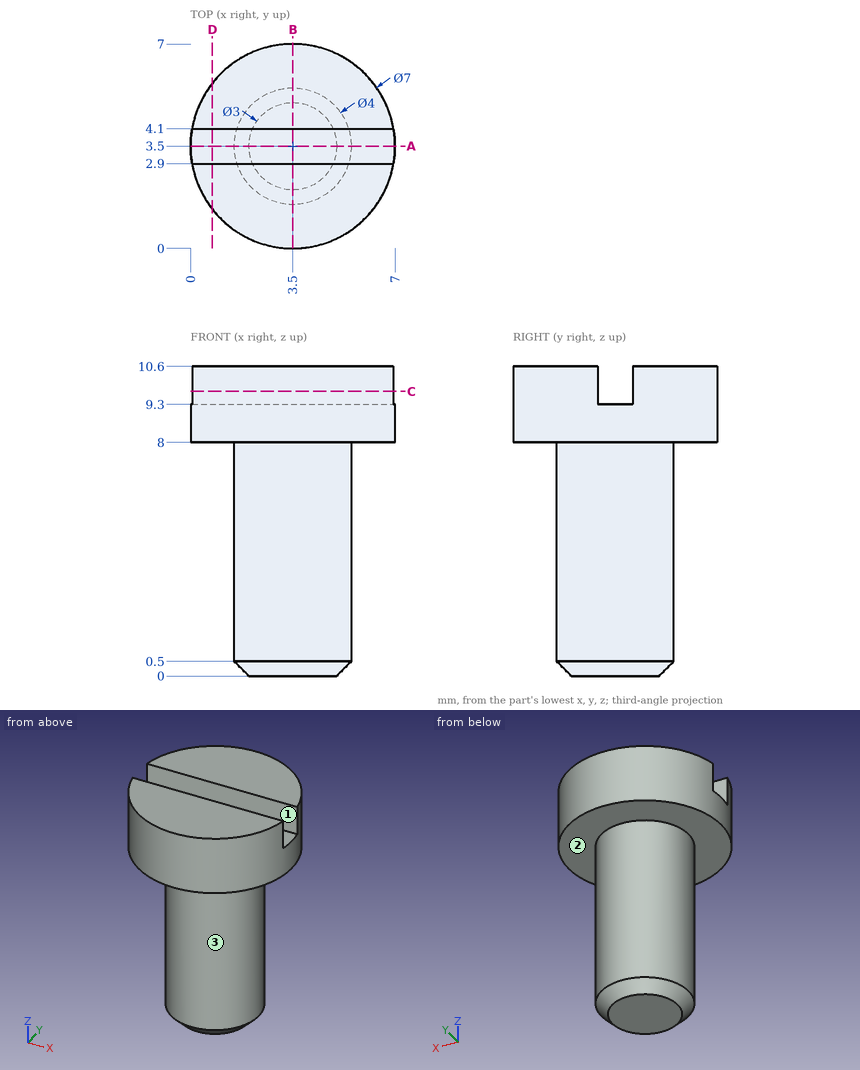
Job drawing, mm, ordinate dimensions from the low corner. One solid piece. Give positions to 0.01 mm unless a question says otherwise; leave off trailing zeros. Write each loop counter-clockwise with the first axis right and the second up, starting at its lowest first coordinate (ties: lowest second). Pieces come first, ordered by that corner, then holes. Notation, with made-up numbers: M -29,12 L -19,12 A35 ccw -19,45 Z; hole C 15,89 d5. An arc over 180 degrees is marked long. One line per item, written item: value. Start each with the question number.
Q1. Saw through at A-A, the plane y = 3.5. Write the cut outline in (x, z), plus the area to 4 significant figures.
Q2. Saw through at C-C, the plane z = 9.75. Write the cut outline in (x, y), plus the area to 3 significant figures.
Q3. Saw through at D-D, the plane x = 0.75. Write the cut outline in (y, z), plus the area to 3 significant figures.
Q4. Drop flat-ended pins along their axis: pin 1 Ø1 at (y, z) = (2, 5.5) entering from +X; pin 2 Ø1.4 at (x, z) = (5, 10.5) entering from +Y; pin 3 Ø4 at (y, z) = (6, 3) entering from -X. Give the stop position or say it passes through.
Q5. Probe probe 1 along Z at (x, y) = (6, 4.25); probe 2 along Z at (x, y) = (3.25, 3.5); probe 3 along Y at (x, z) = (3, 7). List the from-to ranges inside material, lowest first. Write a range as [from, to].
Q6. Two-plate mould, pull along Y, no slides. Class the marked faces 1, 2 and 3: +Y half, -Y half, draft (parallel to the pull), parting line (faces both ways), or undercut.
Q7. Saw through at B-B, the plane x = 3.5. Write the cut outline in (y, z), plus the area to 3 significant figures.
Output values:
1. outline: M 0,8 L 1.5,8 L 1.5,0.5 L 2,0 L 5,0 L 5.5,0.5 L 5.5,8 L 7,8 L 7,9.3 L 0,9.3 Z
1. area: 40.85 mm²
2. outline: M 0.05,2.9 A3.5 ccw 6.95,2.9 Z; M 0.05,4.1 L 6.95,4.1 A3.5 ccw Z
2. area: 30.1 mm²
3. outline: M 1.33,8 L 5.67,8 L 5.67,10.6 L 4.1,10.6 L 4.1,9.3 L 2.9,9.3 L 2.9,10.6 L 1.33,10.6 Z
3. area: 9.70 mm²
4. pin 1: stops at x = 5.23
4. pin 2: stops at y = 6.91
4. pin 3: stops at x = 1.56
5. probe 1: z = [8, 10.6]
5. probe 2: z = [0, 9.3]
5. probe 3: y = [1.56, 5.44]
6. face 1: undercut
6. face 2: draft
6. face 3: parting line
7. outline: M 0,8 L 1.5,8 L 1.5,0.5 L 2,0 L 5,0 L 5.5,0.5 L 5.5,8 L 7,8 L 7,10.6 L 4.1,10.6 L 4.1,9.3 L 2.9,9.3 L 2.9,10.6 L 0,10.6 Z
7. area: 48.4 mm²
